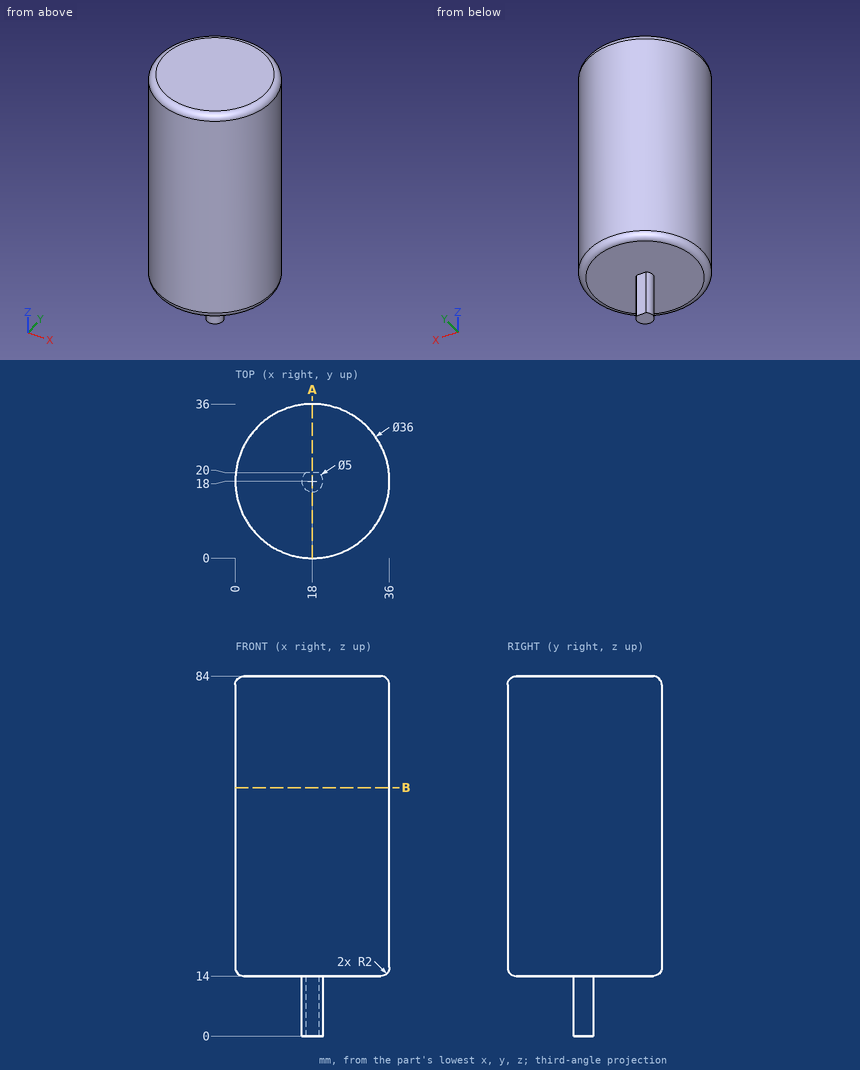
Here's the drawing with two shaded views (mm, measured from the low corner). I have some questions. Coordinates: 2 decimals unless noted, no trailing zeros. Write each loop counter-clockwise with the first axis right and the second up, starting at its lowest first coordinate (ties: lowest second). Pieces come first, ordered by that corner, then holes. Notation, with made-up numbers: (-24.75, 34.25) -> (-10.75, 34.25) arc R14 ccw to (-10.75, 48.25) -> close; hole circle Ø1 at (50.25, 53). An arc over 180 degrees is marked (long way). Answer as CSV lines item,"result".
1) If I drill on line 1 (Z direction, x = 27, y = 28.5); line 2 (X direction, y = 18.5, z = 41.5); line 3 (Y direction, x = 3, z = 26), over which ranges is the centre line in solid material (lowest first)? Write a range as from..to.
Check result:
line 1,"14..84"
line 2,"0.01..35.99"
line 3,"8.05..27.95"
2) Will these pins go through, and if not, where does the flat tip stop? P1, Ø1, axis at y = 22.5, z = 38.5, coming from the -X side; P2, Ø12, axis at x = 22.5, z = 16, coming from the +Y side; P3, Ø1, axis at x = 16.5, y = 9, coming from the -Z side.
Check result:
P1,"x = 0.45"
P2,"y = 36"
P3,"z = 14"
3) If we section it at A-A on x = 18: Please give me the cut outline in (y, z).
Check result:
outline,"(0, 16) arc R2 ccw to (2, 14) -> (15.5, 14) -> (15.5, 0) -> (20, 0) -> (20, 14) -> (34, 14) arc R2 ccw to (36, 16) -> (36, 82) arc R2 ccw to (34, 84) -> (2, 84) arc R2 ccw to (0, 82) -> close"
4) If we section it at B-B on z = 58: Please give me the cut outline in (x, y), then the cut area to 3 significant figures.
Check result:
outline,"circle Ø36 at (18, 18)"
area,"1,020 mm²"
